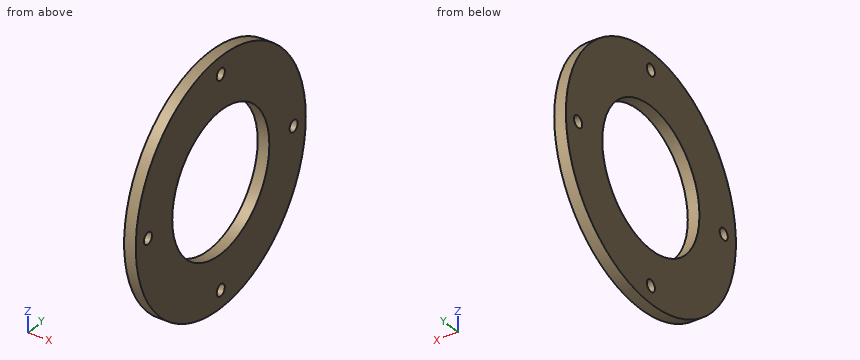
Autodesk Inventor part; units mm, degrees
ref_plane "YZ Plane" through (0, 0, 0) normal (1, 0, 0) x (0, 1, 0)
ref_plane "XZ Plane" through (0, 0, 0) normal (0, 1, 0) x (-1, 0, 0)
ref_plane "XY Plane" through (0, 0, 0) normal (0, 0, 1) x (1, 0, 0)
sketch "Sketch3" plane through (0, 0, 0) normal (1, 0, 0) x (0, 1, 0)
  circle A0 centre (0, 0) radius 66.675
  circle A1 centre (0, -57.15) radius 3.175
  circle A2 centre (57.15, 0) radius 3.175
  circle A3 centre (0, 57.15) radius 3.175
  circle A4 centre (-57.15, 0) radius 3.175
  line L0 (0, 0) -> (79.9058, 0)
  circle A5 centre (0, 0) radius 38.1
  dimension "d13" = 133.35
  dimension "d14" = 6.35
  dimension "d17" = 360
  dimension "d19" = 57.15
  dimension "d20" = 76.2
extrude "Extrusion3" add sketch "Sketch3" along normal blind 6.35
properties part number "BearingAdapter"
Geometry check sheet. Reference: the model listing, model coordinates, mm. Round coordinates to 2 decimals unless told otherwise and drop trailing zeros. Loops run counter-clockwise (first coordinate to the right, second up) from the corner with the lowest first, then second, coordinate; pieces in that order, holes last.
Item 1: Cross-section at D-D on x = 4.5. Record the boundary of the cut face in (y, z) (3 decimals), then the cut area to 3 significant figures.
Item 2: Thickness scan on line 1 (Z direction, x = 3.25, y = 0) (3 decimals); line 2 (Z direction, x = 2, y = 60); line 3 (Y direction, x = 1, z = -10). Record the ranges inside material, lowest first.
Item 3: Gauge pin test, flat ends, axial feed: pin 1 (7.5 mm diameter, centred on y = 0, z = 57.15, fed in from -X); pin 2 (5 mm diameter, centred on y = -57.15, z = 0, fed in from -X). Record the tip position at first contact, or that the pin passes through.
Item 4: Cross-section at A-A on z = 0. Record the boundary of the cut face in (x, y) (3 decimals), then the cut area to 3 significant figures.
Item 5: Cross-section at C-C on y = 57.15. Record the boundary of the cut face in (x, z) (3 decimals).
Answer sheet:
1. outline: circle Ø133.35 at (0, 0); hole circle Ø6.35 at (-57.15, 0); hole circle Ø76.2 at (0, 0); hole circle Ø6.35 at (0, -57.15); hole circle Ø6.35 at (0, 57.15); hole circle Ø6.35 at (57.15, 0)
1. area: 9,280 mm2
2. line 1: z = -66.675 to -60.325, -53.975 to -38.1, 38.1 to 53.975, 60.325 to 66.675
2. line 2: z = -29.08 to -1.4, 1.4 to 29.08
2. line 3: y = -65.92 to -36.76, 36.76 to 65.92
3. pin 1: stops at x = 0
3. pin 2: passes through
4. outline: (0, -66.675) - (6.35, -66.675) - (6.35, -60.325) - (0, -60.325) - close; (0, -53.975) - (6.35, -53.975) - (6.35, -38.1) - (0, -38.1) - close; (0, 38.1) - (6.35, 38.1) - (6.35, 53.975) - (0, 53.975) - close; (0, 60.325) - (6.35, 60.325) - (6.35, 66.675) - (0, 66.675) - close
4. area: 282 mm2
5. outline: (0, -34.343) - (6.35, -34.343) - (6.35, -3.175) - (0, -3.175) - close; (0, 3.175) - (6.35, 3.175) - (6.35, 34.343) - (0, 34.343) - close
